Input: dimensioned drawing with shaded views. Units: mm. Origin: part minimum x, y, z. Round coordinates to 2 decimals unless told otherwise and drop trailing zeros. Write each loop counter-clockwise with the first axis right and the second up, starting at its lowest first coordinate (ties: lowest second). Pieces come first, ordered by that corner, then holes. Notation, with made-up numbers: M -28.75,-30 L -21.75,-30 A19 ccw -21.75,-13 Z; hole C 17,-3.5 d1. An arc over 180 degrees is marked long. Use one line per item in the form item = value. Start each with the question number.
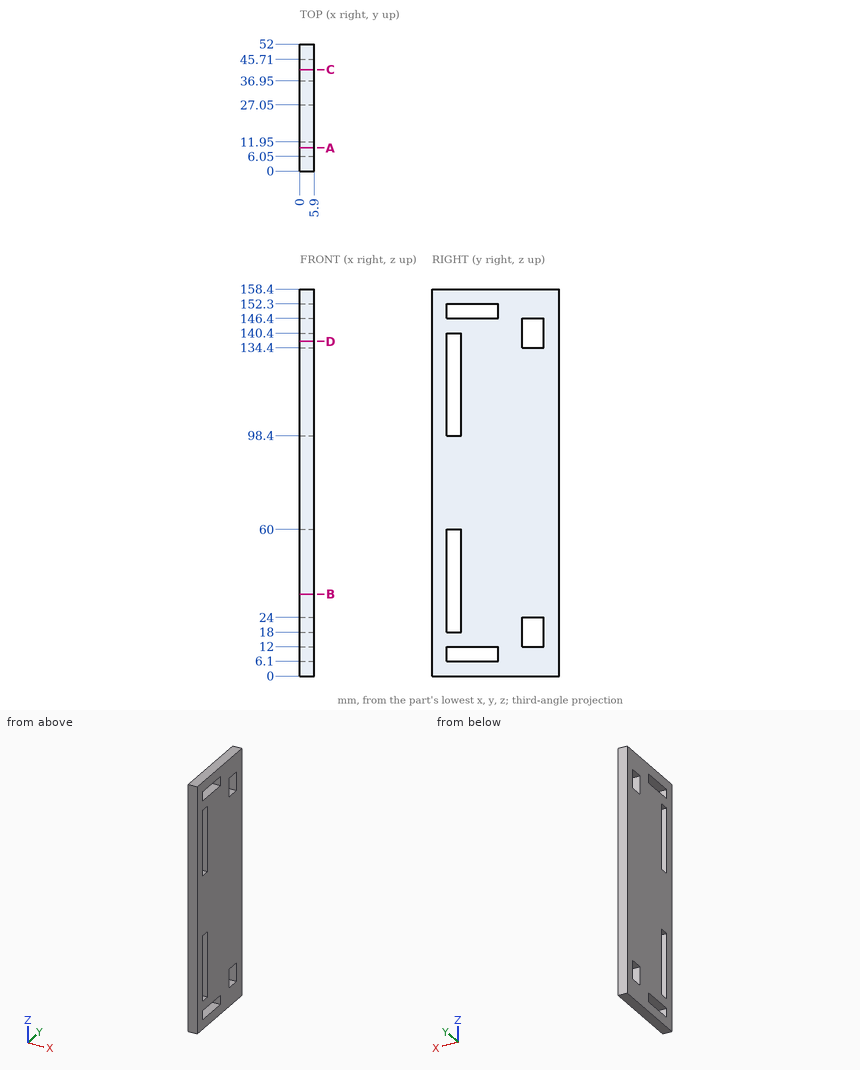
1. Section query C-C (y = 41.5). Return loops of the section in (x, z).
2. Section query B-B (z = 33.5). Return loops of the section in (x, y).
3. Section query A-A (y = 9.5). Return loops of the section in (x, z), then the cut area to 3 significant figures.
4. Section query D-D (z = 137). Return loops of the section in (x, y).
5. Ray query, probe 1 along Y at (x, z) = (2.25, 137.5); probe 2 along Z at (x, y) = (1.95, 12.5); probe 3 along Z at (x, y) = (2.55, 7). Return the intervals inside material, ascending.
Checks:
q1.outline = M 0,0 L 5.9,0 L 5.9,12 L 0,12 Z; M 0,24 L 5.9,24 L 5.9,134.4 L 0,134.4 Z; M 0,146.4 L 5.9,146.4 L 5.9,158.4 L 0,158.4 Z
q2.outline = M 0,0 L 5.9,0 L 5.9,6.05 L 0,6.05 Z; M 0,11.95 L 5.9,11.95 L 5.9,52 L 0,52 Z
q3.outline = M 0,0 L 5.9,0 L 5.9,6.1 L 0,6.1 Z; M 0,12 L 5.9,12 L 5.9,18 L 0,18 Z; M 0,60 L 5.9,60 L 5.9,98.4 L 0,98.4 Z; M 0,140.4 L 5.9,140.4 L 5.9,146.4 L 0,146.4 Z; M 0,152.3 L 5.9,152.3 L 5.9,158.4 L 0,158.4 Z
q3.area = 369 mm^2
q4.outline = M 0,0 L 5.9,0 L 5.9,6.05 L 0,6.05 Z; M 0,11.95 L 5.9,11.95 L 5.9,36.95 L 0,36.95 Z; M 0,45.71 L 5.9,45.71 L 5.9,52 L 0,52 Z
q5.probe_1 = 0 to 6.05, 11.95 to 36.95, 45.71 to 52
q5.probe_2 = 0 to 6.1, 12 to 146.4, 152.3 to 158.4
q5.probe_3 = 0 to 6.1, 12 to 18, 60 to 98.4, 140.4 to 146.4, 152.3 to 158.4
